Verification items for the finished model (mm, model axes). A direction names the side the tool comes from. Round coordinates to 2 decimals unless told otherwise and drop trailing zeros. Order: outer loops, then holes, each group sorted by start corner. A loop starts at its lowest first (then second) coordinate and runs counter-clockwise, first axis right, second up. Notation, with made-up numbers: M -39.75,-3 L 8.25,-3 A14 ccw 8.25,2 Z; hole C 50,-19.5 d9. An arc over 180 degrees is marked long. Use CSV: the item, a comma, the result in double quotes. Start each with the question number.
Q1. Sectioned sample at B-B (y = 196). State how many separate pieces and enclosed holes the cut face has, and give its area (3 significant figures).
Q2. Sectioned sample at A-A (z = 5). Enter the section's corners in (x, y), and give its area (3 significant figures).
Q3. Gauge pin test, flat ends, axial feed: pin 1 Ø5 at (x, z) = (-6.5, -1) entering from +Y; pin 2 Ø5 at (y, z) = (193.5, -5.5) entering from +X; pin 3 Ø1.5 at (y, z) = (170.5, 0.5) entering from +X. Record the tip position at first contact, or that the pin passes through.
Q4. Scan lines: line 1 (X direction, y = 183, z = 5); line 2 (X direction, y = 178, z = 5); line 3 (Z direction, x = -5.75, y = 181). Record each from-to range of solid material in increasing order.
Q5. Mould release check, pull along Y, two halves, no side actions. Record for faces 4 (the face through (-8, 182, 7.6)), 5 (the face through (-6.692, 165.492, -0.729)), 6 (the face through (-4.09, 182.63, -1.58)), 7 (the face through (-0.795, 182.972, -2.334)): +Y half, -Y half, draft (parallel to the pull), parting line (faces both ways), or undercut.
Q6. Set-up check for faces 1 (the face through (-8.215, 195.851, -0.43)), 2 (the face through (-11.397, 195.521, -0.43)), 3 (the face through (-7.972, 166.369, 0.661)): record each of +Z, -Z, +X, -X, +Y, -Y from which the full face is reachable in a straight line by a thin tool's end or side.
Q7. Sectioned sample at C-C (z = -5.5). Enter the section's corners in (x, y).
```python
from build123d import *

# Parameters (mm, degrees)
SKETCH3_R               = 8
BOSS_EXTRUDE1_DEPTH     = 30.735789474
CUT_EXTRUDE1_DEPTH      = 12.15350101
CUT_EXTRUDE1_DEPTH_BACK = 12.15350101
BOSS_EXTRUDE2_DEPTH     = 1.2
CUT_EXTRUDE2_DEPTH      = 1.6
SKETCH8_R               = 1.4
SKETCH8_R_2             = 1.6
CUT_EXTRUDE3_DEPTH      = 2.64160469
CUT_EXTRUDE3_DEPTH_BACK = 35.078782599
CUT_EXTRUDE4_DEPTH      = 35.078782599


with BuildPart() as part:
    # Sketch3 → Boss-Extrude1 (new body)
    with BuildSketch(Plane(origin=(-20.344467381, 196.178792599, 0), x_dir=(-0.994665758, -0.103150523, 0), z_dir=(0.103150523, -0.994665758, 0))):
        with Locations((-10.431405186, 0)):
            Circle(SKETCH3_R)
    extrude(amount=BOSS_EXTRUDE1_DEPTH)

    # Sketch4 → Cut-Extrude1 (cut, two sides)
    with BuildSketch(Plane(origin=(10.375761543, 1.076004901, 0), x_dir=(0.103150523, -0.994665758, 0), z_dir=(-0.994665758, -0.103150523, 0))) as cut_extrude1_sk:
        Polygon((-197.230869842, 0), (-189.230869842, 8), (-197.230869842, 8), align=None)
        Polygon((-174.495080368, 8), (-166.495080368, 8), (-166.495080368, 0), align=None)
    extrude(amount=CUT_EXTRUDE1_DEPTH, mode=Mode.SUBTRACT)
    extrude(cut_extrude1_sk.sketch, amount=-CUT_EXTRUDE1_DEPTH_BACK, mode=Mode.SUBTRACT)

    # Sketch5 → Boss-Extrude2 (add, symmetric)
    with BuildSketch(Plane(origin=(10.375761543, 1.076004901, 0), x_dir=(0.103150523, -0.994665758, 0), z_dir=(-0.994665758, -0.103150523, 0))):
        with BuildLine():
            Line((-166.495080368, -2.8), (-164.070209238, 1.4))
            ThreePointArc((-164.070209238, 1.4), (-166.12960703, 2.776045612), (-168.474979356, 1.979898987))
            Line((-168.474979356, 1.979898987), (-166.495080368, 0))
            Line((-166.495080368, 0), (-166.495080368, -2.8))
        make_face()
    extrude(amount=BOSS_EXTRUDE2_DEPTH, both=True)

    # Sketch7 → Cut-Extrude2 (cut, symmetric)
    with BuildSketch(Plane(origin=(10.375761543, 1.076004901, 0), x_dir=(0.103150523, -0.994665758, 0), z_dir=(-0.994665758, -0.103150523, 0))):
        with BuildLine():
            Line((-194.968128142, 2.2627417), (-197.230869842, 0))
            Line((-197.230869842, 0), (-197.230869842, -3.2))
            ThreePointArc((-197.230869842, -3.2), (-194.274455338, -1.224586984), (-194.968128142, 2.2627417))
        make_face()
    extrude(amount=CUT_EXTRUDE2_DEPTH, both=True, mode=Mode.SUBTRACT)

    # Sketch8 → Cut-Extrude3 (cut, two sides)
    with BuildSketch(Plane(origin=(-20.344467381, 196.178792599, 0), x_dir=(0.994665758, 0.103150523, 0), z_dir=(-0.103150523, 0.994665758, 0))) as cut_extrude3_sk:
        with Locations((10.431405186, -5.5)):
            Circle(SKETCH8_R)
        with Locations((6.831405186, 3)):
            Circle(SKETCH8_R_2)
        with Locations((14.031405186, 3)):
            Circle(SKETCH8_R_2)
    extrude(amount=CUT_EXTRUDE3_DEPTH, mode=Mode.SUBTRACT)
    extrude(cut_extrude3_sk.sketch, amount=-CUT_EXTRUDE3_DEPTH_BACK, mode=Mode.SUBTRACT)

    # Sketch9 → Cut-Extrude4 (cut, through all)
    with BuildSketch(Plane(origin=(-20.344467381, 196.178792599, 0), x_dir=(0.994665758, 0.103150523, 0), z_dir=(-0.103150523, 0.994665758, 0))):
        with BuildLine():
            Line((7.933405986, 7.6), (12.929404385, 7.6))
            ThreePointArc((12.929404385, 7.6), (10.431405186, 8), (7.933405986, 7.6))
        make_face()
        with BuildLine():
            Line((7.933405986, -7.6), (12.929404385, -7.6))
            ThreePointArc((12.929404385, -7.6), (10.431405186, -8), (7.933405986, -7.6))
        make_face()
    extrude(amount=-CUT_EXTRUDE4_DEPTH, mode=Mode.SUBTRACT)


solid = part.part
```
Verdict:
1,separate pieces,"1"
1,enclosed holes,"2"
1,area,"90.1 mm²"
2,outline,"M -15.66,191.64 L -13.53,171.01 L -8.61,171.52 L -10.75,192.15 Z; M -8.15,192.42 L -6.01,171.79 L -1.1,172.3 L -3.24,192.93 Z"
2,area,"205 mm²"
3,pin 1,"stops at y = 197.87"
3,pin 2,"stops at x = -2.09"
3,pin 3,"stops at x = 0.92"
4,line 1,"x = -14.77 to -9.81, -7.18 to -2.21"
4,line 2,"x = -14.25 to -9.29, -6.66 to -1.69"
4,line 3,"z = -7.59 to -4.18, -1.82 to 7.59"
5,face 4,"draft"
5,face 5,"-Y half"
5,face 6,"undercut"
5,face 7,"+Y half"
6,face 1,"none"
6,face 2,"+Y"
6,face 3,"+Z, -Y"
7,outline,"M -15.75,196.66 L -12.58,166.08 L -1.02,167.28 L -4.19,197.85 Z"
